Drawing for the job (mm, zero at the part's lowest x, y, z). A direction names the side the tool comes from. Round coordinates to 2 decimals unless told otherwise and drop trailing zeros. Order: outer loops, then holes, each group sorted by start corner. A loop starts at its lowest first (then second) coordinate and runs counter-clockwise, first axis right, second up. Notation, with made-up numbers: (26.5, 83) - (54.5, 83) arc R15 cw to (54.5, 112) - close; hole circle Ø2 at (46, -39.75). An arc over 180 degrees is marked (long way). Put each result on its own line as item: value. Start each with the question number.
Item 1: Saw through at A-A on y = 41. List the corners of the cut face in (x, z).
Item 2: Which spindle directions (+Z, -Z, +X, -X, +Y, -Y) get a long thin tool onto all of the face, cutting with end or side? Do the marked faces 1 and 2. Say none if no direction does.
Item 3: Saw through at B-B on x = 22. List the corners of the cut face in (y, z).
Item 4: Pin check, flat tips, straight feed: pin 1 Ø6 at (x, y) = (34.5, 6.5) entering from -Z; pin 2 Ø19 at (x, z) = (17.5, 24) entering from -Y. Stop position of each tip, or through.
Item 5: Saw through at C-C on x = 15.5. List the corners of the cut face in (y, z), plus the area to 3 significant figures.
Item 6: Saw through at D-D on z = 31. List the corners of the cut face in (x, y).
Item 7: Probe probe 1 along Z at (x, y) = (25.4, 48.25); probe 2 along X at (y, z) = (41.75, 31.75); probe 3 along Z at (x, y) = (39.5, 9.5). List the from-to ranges inside material, lowest first.
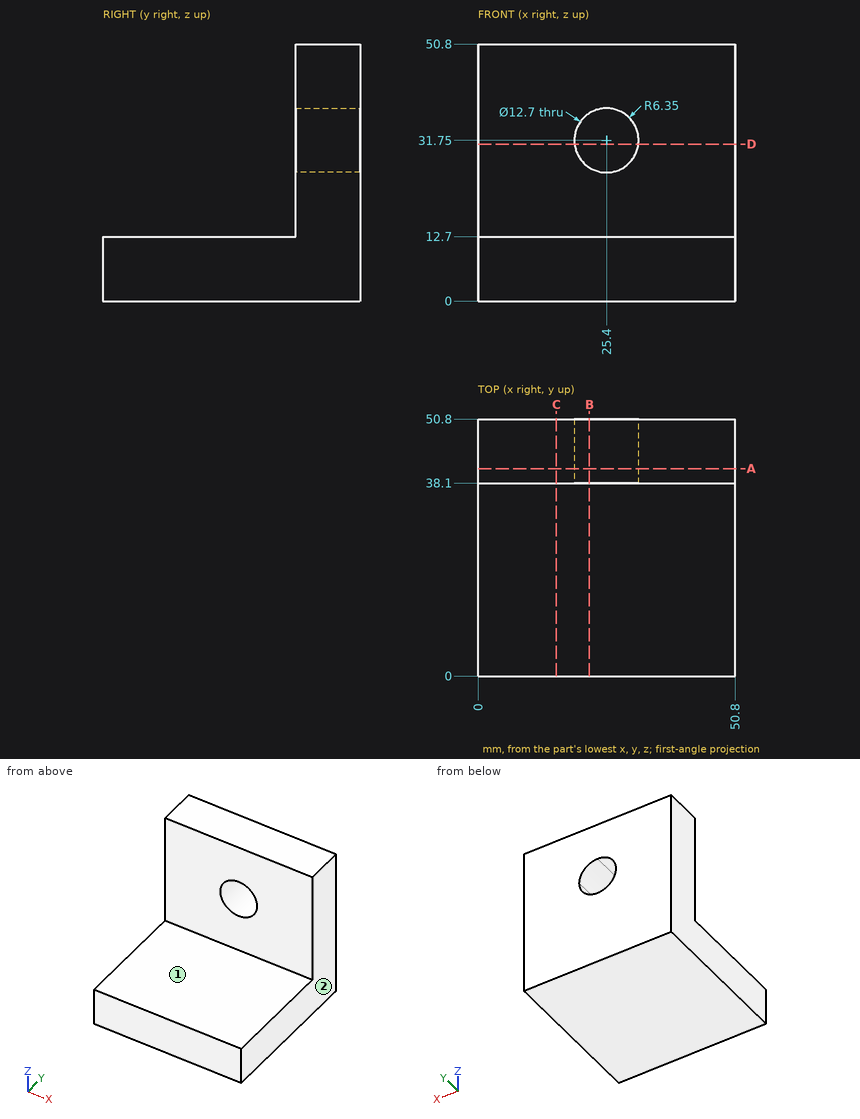
Results found:
1. outline: (0, 0) - (50.8, 0) - (50.8, 50.8) - (0, 50.8) - close; hole circle Ø12.7 at (25.4, 31.75)
2. face 1: +Z, +X, -X, -Y
2. face 2: +Z, -Z, +X, +Y, -Y
3. outline: (0, 0) - (50.8, 0) - (50.8, 26.39) - (38.1, 26.39) - (38.1, 12.7) - (0, 12.7) - close; (38.1, 37.11) - (50.8, 37.11) - (50.8, 50.8) - (38.1, 50.8) - close
4. pin 1: stops at z = 0
4. pin 2: stops at y = 38.1
5. outline: (0, 0) - (50.8, 0) - (50.8, 50.8) - (38.1, 50.8) - (38.1, 12.7) - (0, 12.7) - close
5. area: 1,130 mm²
6. outline: (0, 38.1) - (19.09, 38.1) - (19.09, 50.8) - (0, 50.8) - close; (31.71, 38.1) - (50.8, 38.1) - (50.8, 50.8) - (31.71, 50.8) - close
7. probe 1: z = 0 to 25.4, 38.1 to 50.8
7. probe 2: x = 0 to 19.05, 31.75 to 50.8
7. probe 3: z = 0 to 12.7
